from build123d import *

# Parameters (mm, degrees)
SKETCH_1_R          = 2
SKETCH_1_R_2        = 1.75
EXTRUDE_1_DEPTH     = 25
SKETCH_1_3_R        = 1.75
EXTRUDE_2_DEPTH     = 20
SKETCH_2_R          = 3.5
EXTRUDE_3_DEPTH     = 4
CUT_EXTRUDE_1_DEPTH = 3


with BuildPart() as part:
    # Sketch 1 → Extrude 1 (new body)
    with BuildSketch(Plane(origin=(0, 0, 0), x_dir=(1, 0, 0), z_dir=(0, 1, 0))):
        with Locations(Location((0, 0, 0), (0, 0, 270))):
            Circle(SKETCH_1_R)
        Circle(SKETCH_1_R_2, mode=Mode.SUBTRACT)
        Circle(SKETCH_1_R_2)
    extrude(amount=EXTRUDE_1_DEPTH)

    # Sketch 1_3 → Extrude 2 (add)
    with BuildSketch(Plane(origin=(0, 0, 0), x_dir=(1, 0, 0), z_dir=(0, 1, 0))):
        with Locations(Location((0, 0, 0), (0, 0, 270))):
            Circle(SKETCH_1_3_R)
    extrude(amount=-EXTRUDE_2_DEPTH)

    # Sketch 2 → Extrude 3 (add)
    with BuildSketch(Plane(origin=(0, 25, 0), x_dir=(1, 0, 0), z_dir=(0, 1, 0))):
        with Locations(Location((0, 0, 0), (0, 0, 270))):
            Circle(SKETCH_2_R)
    extrude(amount=EXTRUDE_3_DEPTH)

    # Sketch 3 → Cut-Extrude 1 (cut)
    with BuildSketch(Plane(origin=(0, 29, 0), x_dir=(1, 0, 0), z_dir=(0, 1, 0))):
        Polygon((1.22041658, -0.939246172), (1.423619335, 0.587288675), (0.203202756, 1.526534847), (-1.22041658, 0.939246172), (-1.423619335, -0.587288675), (-0.203202756, -1.526534847), align=None)
    extrude(amount=-CUT_EXTRUDE_1_DEPTH, mode=Mode.SUBTRACT)


solid = part.part
Model file for the job. Use its own axes, mm. A direction names the side the tool comes from. Coordinates: 2 decimals unless noted, no trailing zeros. Loops run counter-clockwise (first coordinate to the right, second up) from the corner with the lowest first, then second, coordinate; pieces in that order, holes last. Notation, with made-up numbers: (12.25, 62) -> (22.25, 62) arc R21 cw to (22.25, 89) -> close; hole circle Ø7 at (17.25, 3). An arc over 180 degrees is marked (long way). Use one line per item in the form item = value. Start each with the question number.
(1) Cut at D-D on y = -0.5. Give the cut face in (x, z), and give its area (3 significant figures).
(2) Cut at B-B on x = 0.75. Give the cut face in (y, z), and give its area (3 significant figures).
(3) Tool access for faces 1 (the flat face through (0, -20, 0)), 2 (the flat face through (0.82, 27.52, -1.05)), 3 (the cylindrical face through (-1.71, -9.86, -0.38)): list every direction of +Z, -Z, +X, -X, +Y, -Y with a clear straight run to the whole face (end or side of a thin tool).
(4) Pull direction Z, two halves, no side cores. Call faces 4 (the flat face through (0, 29, 2)), 5 (the cylindrical face through (-3.417, 26.972, -0.759)), 6 (the flat face through (-1.32, 27.52, -0.19)): pulls with the +Z half, pulls with the -Z half, needs draft (parallel to the pull), parting line crosses it, or undercut.
(5) Probe probe 1 along Y at (x, z) = (2.25, 0.5); probe 2 along Y at (x, z) = (-0.5, -0.5); probe 3 along X at (y, z) = (-3.5, -1.25). List the from-to ranges inside material, lowest first. Write a range as from..to.
(6) Cut at C-C on y = 7.5. Give the cut face in (x, z), and give its area (3 significant figures).
(7) Flat gauge pins, fed straight in: pin 1 (0.9 mm diameter, centred on x = 0.5, z = 0.5, fed in from +Y); pin 2 (1.5 mm diameter, centred on y = 3.5, z = 0.5, fed in from +X). Where does each tip first touch, or does it go through?
(8) Cut at A-A on z = 0. Give the cut face in (x, y), and give its area (3 significant figures).
Values:
q1.outline = circle Ø3.5 at (0, 0)
q1.area = 9.62 mm2
q2.outline = (-20, -1.58) -> (0, -1.58) -> (0, -1.85) -> (25, -1.85) -> (25, -3.42) -> (29, -3.42) -> (29, -1.11) -> (26, -1.11) -> (26, 1.13) -> (29, 1.13) -> (29, 3.42) -> (25, 3.42) -> (25, 1.85) -> (0, 1.85) -> (0, 1.58) -> (-20, 1.58) -> close
q2.area = 177 mm2
q3.face_1 = +Z, -Z, +X, -X, -Y
q3.face_2 = +Y
q3.face_3 = -Y
q4.face_4 = needs draft
q4.face_5 = parting line crosses it
q4.face_6 = undercut
q5.probe_1 = 25..29
q5.probe_2 = -20..26
q5.probe_3 = -1.22..1.22
q6.outline = circle Ø4 at (0, 0)
q6.area = 12.6 mm2
q7.pin_1 = 26
q7.pin_2 = 2
q8.outline = (-3.5, 25) -> (-2, 25) -> (-2, 0) -> (-1.75, 0) -> (-1.75, -20) -> (1.75, -20) -> (1.75, 0) -> (2, 0) -> (2, 25) -> (3.5, 25) -> (3.5, 29) -> (1.35, 29) -> (1.35, 26) -> (-1.35, 26) -> (-1.35, 29) -> (-3.5, 29) -> close
q8.area = 190 mm2
